The drawing under review shows one solid part. Ordinate dimensions are in mm from its lowest x, y, z. Coordinates: 2 decimals unless noted, no trailing zeros. Order: outer loops, then holes, each group sorted by start corner. A loop starts at its lowest first (then second) coordinate and runs counter-clockwise, first axis right, second up. Notation, with made-up numbers: (68, -18.5) - (84, -18.5) arc R30 cw to (84, 6.5) - close; hole circle Ø10 at (6.25, -25.75). An arc over 180 degrees is marked (long way). Write item = value, one per line. Start each with the question number.
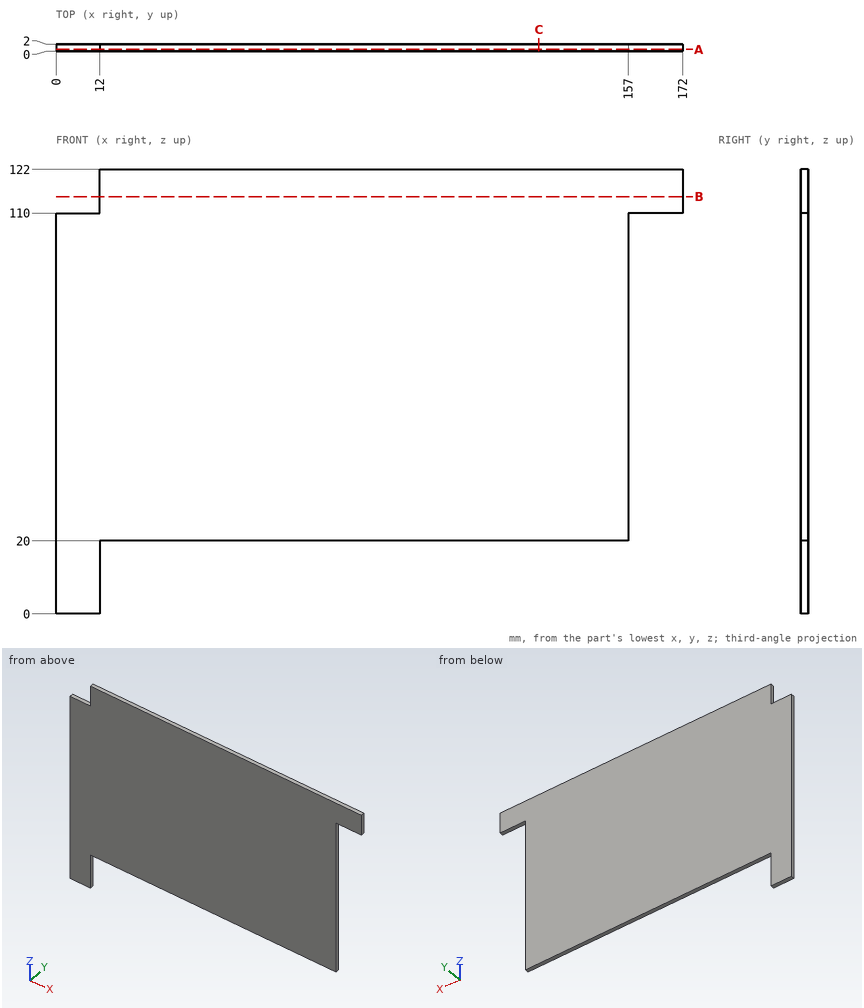
Item 1: For line 1 (Z direction, x = 22.5, y = 1.15); line 2 (X direction, y = 1.1, z = 91), list the stretches that pass through material, from the lowest coordinate up.
Item 2: Add section A-A on y = 0.55. Give the boundary of the cut face in (x, z), plus the area to 3 significant figures.
Item 3: Add section C-C on x = 132.5. Give the boundary of the cut face in (y, z), plus the area to 3 significant figures.
Item 4: Add section B-B on z = 114.5. Give the boundary of the cut face in (x, y).
Item 5: For P1, Ø1, axis at y = 1, z = 113, coming from the -X side; P2, Ø1, axis at x = 70.5, y = 1.5, coming from the -Z side; P3, Ø0.6, axis at y = 1.5, z = 15, coming from the +X side; P4, Ø2, axis at x = 123.5, z = 18.5, coming from the -Y side, all flat-tipped, find the tip position at first contact; note any pin that passes through.
Worked out:
q1.line_1 = 20 to 122
q1.line_2 = 0 to 157
q2.outline = (0, 0) - (12, 0) - (12, 20) - (157, 20) - (157, 110) - (172, 110) - (172, 122) - (12, 122) - (12, 110) - (0, 110) - close
q2.area = 16,300 mm2
q3.outline = (0, 20) - (2, 20) - (2, 122) - (0, 122) - close
q3.area = 204 mm2
q4.outline = (12, 0) - (172, 0) - (172, 2) - (12, 2) - close
q5.P1 = 12
q5.P2 = 20
q5.P3 = 12
q5.P4 = through
